```python
from build123d import *

# Parameters (mm, degrees)
SKETCH1_R                         = 26.416
BOSS_EXTRUDE1_DEPTH               = 201.549
SKETCH8_R                         = 17.4244
BOSS_EXTRUDE2_DEPTH               = 25.4
CUT_EXTRUDE1_START                = -22.352
CUT_EXTRUDE1_DEPTH                = 22.352
SKETCH16_R                        = 4.826
CUT_EXTRUDE2_DEPTH                = 232.290745898
BOSS_EXTRUDE3_START               = 20.574
SKETCH17_R                        = 17.4244
BOSS_EXTRUDE3_DEPTH               = 20.574
SKETCH20_R                        = 10.033
CUT_EXTRUDE3_DEPTH                = 23.749
SKETCH22_R                        = 23.241
CUT_EXTRUDE4_DEPTH                = 281.051
F_1_4_NPT_TAPPED_HOLE3_AT_2_COUNT = 2
F_1_4_NPT_TAPPED_HOLE3_AT_2_PITCH = 372.618


# Read off the part's stored shape, not the designer's step: 1-1/4-7 Machine Threads Stud1, 1-1/4-12 Machine Threads Stud1
with BuildPart() as part:
    # Sketch1 → Boss-Extrude1 (new, symmetric)
    with BuildSketch(Plane(origin=(0, 0, 0), x_dir=(0, 0, -1), z_dir=(1, 0, 0))):
        Circle(SKETCH1_R)
    extrude(amount=BOSS_EXTRUDE1_DEPTH, both=True)

    # Sketch8 → Boss-Extrude2 (add)
    with BuildSketch(Plane.ZY.offset(201.549)):
        Circle(SKETCH8_R)
    extrude(amount=BOSS_EXTRUDE2_DEPTH)

    # 1-1/4-7 Machine Threads Stud1 outline → 1-1/4-7 Machine Threads Stud1 (revolve, cut)
    with BuildSketch(Plane.YX):
        Polygon((13.71473, -226.949), (17.4244, -226.949), (17.4244, -204.597), (15.875, -204.597), (15.875, -224.78873), align=None)
    revolve(axis=Axis((0, 0, 0), (1, 0, 0)), mode=Mode.SUBTRACT)

    # Sketch15 → Cut-Extrude1 (cut)
    with BuildSketch(Plane.ZY.offset(226.949).offset(CUT_EXTRUDE1_START)):
        with BuildLine():
            Line((-9.525, 14.59054798), (-9.525, -14.59054798))
            ThreePointArc((-9.525, -14.59054798), (-17.4244, 0), (-9.525, 14.59054798))
        make_face()
        with BuildLine():
            Line((9.525, 14.59054798), (9.525, -14.59054798))
            ThreePointArc((9.525, -14.59054798), (17.4244, 0), (9.525, 14.59054798))
        make_face()
    extrude(amount=CUT_EXTRUDE1_DEPTH, mode=Mode.SUBTRACT)

    # Sketch16 → Cut-Extrude2 (cut, through all)
    with BuildSketch(Plane.XY.offset(9.525)):
        with Locations((-215.773, 0)):
            Circle(SKETCH16_R)
    extrude(amount=-CUT_EXTRUDE2_DEPTH, mode=Mode.SUBTRACT)

    # Sketch17 → Boss-Extrude3 (add)
    with BuildSketch(Plane(origin=(201.549, 0, 0), x_dir=(0, 0, -1), z_dir=(1, 0, 0)).offset(BOSS_EXTRUDE3_START)):
        Circle(SKETCH17_R)
    extrude(amount=-BOSS_EXTRUDE3_DEPTH)

    # Sketch20 → Cut-Extrude3 (cut)
    with BuildSketch(Plane(origin=(222.123, 0, 0), x_dir=(0, 0, -1), z_dir=(1, 0, 0))):
        Circle(SKETCH20_R)
    extrude(amount=-CUT_EXTRUDE3_DEPTH, mode=Mode.SUBTRACT)

    # Sketch22 → Cut-Extrude4 (cut)
    with BuildSketch(Plane(origin=(198.374, 0, 0), x_dir=(0, 0, -1), z_dir=(1, 0, 0))):
        Circle(SKETCH22_R)
    extrude(amount=-CUT_EXTRUDE4_DEPTH, mode=Mode.SUBTRACT)

    # Sketch26 → 1/4 NPT Tapped Hole3 (revolve, cut)
    with BuildSketch(Plane(origin=(-189.611, 0, 26.416), x_dir=(0, -1, 0), z_dir=(1, 0, 0))):
        Polygon((0, 0), (0, 34.299867279), (5.5626, 30.95752), (5.5626, 26.7208), (6.557980564, 26.7208), (7.3580371, 0), align=None)
    f_1_4_npt_tapped_hole3 = revolve(axis=Axis((-189.611, 0, 32.766), (0, 0, -1)), mode=Mode.SUBTRACT)

    # 1/4 NPT Tapped Hole3 at 2: 1/4 NPT Tapped Hole3 ×2
    with Locations(*[(i * F_1_4_NPT_TAPPED_HOLE3_AT_2_PITCH, 0, 0) for i in range(1, F_1_4_NPT_TAPPED_HOLE3_AT_2_COUNT)]):
        add(f_1_4_npt_tapped_hole3, mode=Mode.SUBTRACT)

    # 1-1/4-12 Machine Threads Stud1 outline → 1-1/4-12 Machine Threads Stud1 (revolve, cut)
    with BuildSketch(Plane.YX):
        Polygon((17.4244, 222.123), (14.61516, 222.123), (15.875, 220.86316), (15.875, 204.597), (17.4244, 204.597), align=None)
    revolve(axis=Axis((0, 0, 0), (1, 0, 0)), mode=Mode.SUBTRACT)


solid = part.part
```
The model under review builds one solid part; all positions refer to its coordinate system, in mm. A direction names the side the tool comes from. Give positions to 0.01 mm unless a question says otherwise; leave off trailing zeros. Loops run counter-clockwise (first coordinate to the right, second up) from the corner with the lowest first, then second, coordinate; pieces in that order, holes last. Notation, with made-up numbers: (76, 81.5) -> (133, 81.5) arc R16 ccw to (133, 89.5) -> close; hole circle Ø9 at (45.5, 60.5). An arc over 180 degrees is marked (long way). Use CSV: the item, a comma, the result in double quotes.
1. Machinability: for faces 5 (the face through (-82.677, 0, 0)), 6 (the face through (-214.834, -15.874, 0.143)), 7 (the face through (203.09, 5.23, -16.62)), which of the approach directions +Z, -Z, +X, -X, +Y, -Y give a long, thin tool a straight path to every point of the face, cutting with its end or side? Answer none if there is none.
Result:
face 5,"none"
face 6,"-X, -Y"
face 7,"+X"
2. For P1, Ø6, axis at x = 32, z = -10, coming from the +Y side; P2, Ø2, axis at x = -121.5, y = -12.5, coming from the -Z side; P3, Ø11, axis at x = -220, y = 4.5, coming from the +Z side (3 decimals), all flat-tipped, find the tip position at first contact; note any pin that passes through.
Result:
P1,"stops at y = 25.47"
P2,"stops at z = -23.78"
P3,"stops at z = 9.525"
3. Consider section A-A, the plane x = 78.5. Write out the cut boundary in (y, z).
Result:
outline,"circle Ø52.83 at (0, 0); hole circle Ø46.48 at (0, 0)"
4. The part is to be moulded in two halves that separate along Z. For faces 1 (the face through (-203.05, 5.23, 16.62)), 2 (the face through (222.123, 3, -10)), 3 (the face through (210.415, -9.794, 2.175)), 4 (the face through (-188.668, 0.209, -7.303)), say which applies: +Z half, -Z half, draft (parallel to the pull), parting line (faces both ways), or undercut.
Result:
face 1,"parting line"
face 2,"draft"
face 3,"undercut"
face 4,"+Z half"
5. To check wall thickness, follow probe 1 along X at (y, z) = (13, 3); probe 2 along Y at (x, z) = (122, 0); probe 3 along X at (y, z) = (-3.5, -12). State the ranges of each line that lie inside material, in increasing order. Write a range as from..to.
Result:
probe 1,"x = -226.95..-82.68, 198.37..222.12"
probe 2,"y = -26.42..-23.24, 23.24..26.42"
probe 3,"x = -204.6..-82.68, 198.37..222.12"
6. Consider section B-B, the plane x = -137.5. Write out the cut boundary in (y, z), then the cut area to 3 significant figures.
Result:
outline,"circle Ø52.83 at (0, 0)"
area,"2,190 mm²"
